For this review, take the finished solid that the model builds, in its own axes (mm). A direction names the side the tool comes from. Coordinates: 2 decimals unless noted, no trailing zeros. Write each loop counter-clockwise with the first axis right and the second up, starting at its lowest first coordinate (ties: lowest second). Pieces come first, ordered by that corner, then holes.
1) We need section B-B on z = 2.25. Write out the cut boundary in (x, y).
2) For faces 1 (the face through (0, -51, 0)), 2 (the face through (4.955, -46, 6)), list the 3-axis set-ups (+Z, -Z, +X, -X, +Y, -Y) from which the entire face can be reached by the end or side of a thin tool; tool diameter is ignored.
3) Mouldability with a two-part tool opening along Z and no side actions: class faces 3 (the face through (2.512, 18.726, 2.637)), 4 (the face through (0, -49, 11.176)), 5 (the face through (23.449, -29.844, 5.51)) as pulls with the +Z half, pulls with the -Z half, needs draft (parallel to the pull), parting line crosses it, or undercut.
4) We need section A-A on y = -51. Write out the cut boundary in (x, z), then the cut area to 3 significant figures.
5) We need section C-C on y = 45.5. Write out the cut boundary in (x, z).
6) To check wall thickness, follow line 1 along X through (y, z) = (6, 5.75); line 2 along Y through (x, z) = (-11, 4.75); line 3 along Y through (x, z) = (-11.5, 4.5). State the ranges of each line that lie inside material, in increasing order.
7) Insertion check: P1, Ø6, axis at y = 47, z = 4.5, coming from the -X side; P2, Ø0.8, axis at y = 10, z = 5.5, coming from the +X side; P3, Ø9, axis at x = -20, y = -30, coming from the +Z side. Each pin has a flat end and moves straight along its axis. Give the tip position at first contact, or say it passes through.
from build123d import *

# Parameters (mm, degrees)
F1_DEPTH     = 11.176
F2_T1_DEPTH  = 94.3857913817
F2_T4_ANGLE  = 351.4780510153
F2_T6_ANGLE  = 351.4780510153
F2_T8_ANGLE  = 351.4780510153
F2_T10_ANGLE = 351.4780510153
F3_R         = 3.6792614691
F4_R         = 3.6792614691
F5_R         = 4.3813050742
F6_DEPTH     = 2.286


# Not quite as in the source:
# - a fillet or chamfer that OpenCascade refuses, or shapes differently, is made with other operations: its cross-section is extruded or revolved along the edge and cut away or added


with BuildPart() as f1:
    # F0 (on Top) → F1 (new body)
    with BuildSketch(Plane.XY):
        with BuildLine():
            Line((4.9550826661, 52.6113137603), (0, 64.8532807827))
            Line((0, 64.8532807827), (-4.9550826661, 52.6113137603))
            Line((-4.9550826661, 52.6113137603), (-4.9550826661, -28.7103280425))
            ThreePointArc((-4.9550826661, -28.7103280425), (-9.3272130471, -33.0824584235), (-13.699343428, -28.7103280425))
            ThreePointArc((-13.699343428, -28.7103280425), (-23.4025628963, -29.6754723169), (-15.7396737486, -35.7057377696))
            ThreePointArc((-15.7396737486, -35.7057377696), (-10.5930074953, -38.0719437204), (-4.9550826661, -38.6204943061))
            Line((-4.9550826661, -38.6204943061), (-4.9550826661, -53.7772104144))
            ThreePointArc((-4.9550826661, -53.7772104144), (-6.5397395867, -60.7633924821), (0, -63.687376678))
            ThreePointArc((0, -63.687376678), (6.5397395867, -60.7633924821), (4.9550826661, -53.7772104144))
            Line((4.9550826661, -53.7772104144), (4.9550826661, -38.6204943061))
            ThreePointArc((4.9550826661, -38.6204943061), (10.5930074953, -38.0719437204), (15.7396737486, -35.7057377696))
            ThreePointArc((15.7396737486, -35.7057377696), (23.4025628963, -29.6754723169), (13.699343428, -28.7103280425))
            ThreePointArc((13.699343428, -28.7103280425), (9.3272130471, -33.0824584235), (4.9550826661, -28.7103280425))
            Line((4.9550826661, -28.7103280425), (4.9550826661, 52.6113137603))
        make_face()
    extrude(amount=F1_DEPTH)

    # F2: chamfer of 5.08 on 8 edges, made by hand

    # F2_s2 → F2_t1 (cut)
    with BuildSketch(Plane.XZ.offset(-65.6754633391)):
        Polygon((-4.9550826661, 6.096), (0.1249173339, 11.176), (-4.9550826661, 11.176), align=None)
        Polygon((4.9550826661, 6.096), (-0.1249173339, 11.176), (4.9550826661, 11.176), align=None)
        Polygon((-4.9550826661, 5.08), (0.1249173339, 0), (-4.9550826661, 0), align=None)
        Polygon((4.9550826661, 5.08), (-0.1249173339, 0), (4.9550826661, 0), align=None)
    extrude(amount=F2_T1_DEPTH, mode=Mode.SUBTRACT)

    # F2_s3 → F2_t4 (revolve, cut)
    with BuildSketch(Plane(origin=(-4.0027369728, -26.7129328444, 0), x_dir=(0, 0, 1), z_dir=(-0.1481882745, -0.9889591677, 0))):
        Polygon((5.08, -9.1066364436), (0, -4.0266364436), (0, -9.1066364436), align=None)
    revolve(axis=Axis((9.3272130471, -28.7103280425, 0), (0, 0, -1)), revolution_arc=F2_T4_ANGLE, mode=Mode.SUBTRACT)

    # F2_s5 → F2_t6 (revolve, cut)
    with BuildSketch(Plane(origin=(-4.0027369728, -26.7129328444, 0), x_dir=(0, 0, 1), z_dir=(-0.1481882745, -0.9889591677, 0))):
        Polygon((6.096, -9.1066364436), (11.176, -4.0266364436), (11.176, -9.1066364436), align=None)
    revolve(axis=Axis((9.3272130471, -28.7103280425, 11.176), (0, 0, -1)), revolution_arc=F2_T6_ANGLE, mode=Mode.SUBTRACT)

    # F2_s7 → F2_t8 (revolve, cut)
    with BuildSketch(Plane.XZ.offset(28.7103280425)):
        Polygon((-4.9550826661, 5.08), (0.1249173339, 0), (-4.9550826661, 0), align=None)
    revolve(axis=Axis((-9.3272130471, -28.7103280425, 0), (0, 0, -1)), revolution_arc=F2_T8_ANGLE, mode=Mode.SUBTRACT)

    # F2_s9 → F2_t10 (revolve, cut)
    with BuildSketch(Plane.XZ.offset(28.7103280425)):
        Polygon((-4.9550826661, 6.096), (0.1249173339, 11.176), (-4.9550826661, 11.176), align=None)
    revolve(axis=Axis((-9.3272130471, -28.7103280425, 11.176), (0, 0, -1)), revolution_arc=F2_T10_ANGLE, mode=Mode.SUBTRACT)

    # F3
    f3_edges = [f1.edges().sort_by_distance(p)[0] for p in [
        (-4.955083, -46.198852, 11.176),
    ]]
    fillet(f3_edges, radius=F3_R)

    # F4
    f4_edges = [f1.edges().sort_by_distance(p)[0] for p in [
        (4.955083, -46.198852, 11.176),
        (4.955083, -46.198852, 0),
        (-4.955083, -46.198852, 0),
    ]]
    fillet(f4_edges, radius=F4_R)

    # F5 (on face) → F6 (join)
    with BuildSketch(Plane.XY.offset(11.176)):
        with Locations((0, -58.3839304745)):
            Circle(F5_R)
    extrude(amount=F6_DEPTH)

    # F7: fillet of radius 5.08 on 1 edges, made by hand

    # F7_s1 → F7_t2 (revolve, cut)
    with BuildSketch(Plane.XZ.offset(58.3839304745)):
        with BuildLine():
            ThreePointArc((4.3813050742, 11.176), (2.5483242068, 12.8541314829), (0.1386686298, 13.462))
            Line((0.1386686298, 13.462), (4.3813050742, 13.462))
            Line((4.3813050742, 13.462), (4.3813050742, 11.176))
        make_face()
    revolve(axis=Axis((0, -58.3839304745, 13.462), (0, 0, 1)), mode=Mode.SUBTRACT)


solid = f1.part
Result:
1. outline: (-16.14, -26.38) arc R5.26 ccw (long way) to (-15.74, -35.71) arc R17.04 ccw to (-4.67, -38.6) - (-4.67, -53.57) arc R5.65 ccw to (0, -63.69) arc R5.65 ccw to (4.67, -53.57) - (4.67, -38.6) arc R17.04 ccw to (15.74, -35.71) arc R5.26 ccw (long way) to (16.14, -26.38) arc R7.2 cw (long way) to (2.13, -28.71) - (2.13, 59.6) - (0, 64.85) - (-2.13, 59.6) - (-2.13, -28.71) arc R7.2 cw (long way) to start
2. face 1: -Z, +X, -X, +Y, -Y
2. face 2: +Z, -Z, +X
3. face 3: pulls with the -Z half
3. face 4: pulls with the +Z half
3. face 5: needs draft
4. outline: (-4.96, 3.68) arc R3.68 ccw to (-1.28, 0) - (1.28, 0) arc R3.68 ccw to (4.96, 3.68) - (4.96, 7.5) arc R3.68 ccw to (1.28, 11.18) - (-1.28, 11.18) arc R3.68 ccw to (-4.96, 7.5) - close
4. area: 99.1 mm2
5. outline: (-4.96, 5.08) - (0, 0.12) - (4.96, 5.08) - (4.96, 6.1) - (0, 11.05) - (-4.96, 6.1) - close
6. line 1: x = -4.96 to 4.96
6. line 2: y = -37.96 to -33.1
6. line 3: y = -37.8 to -33.16
7. P1: stops at x = -4.96
7. P2: stops at x = 4.96
7. P3: stops at z = 11.18
